Design review of the part built by this model. Coordinates are the model's own, in mm. A direction names the side the tool comes from. Coordinates: 2 decimals unless noted, no trailing zeros. Order: outer loops, then holes, each group sorted by start corner. A loop starts at its lowest first (then second) coordinate and runs counter-clockwise, first axis right, second up.
from build123d import *

# Parameters (mm, degrees)
CROQUIS2_W                   = 50
CROQUIS2_H                   = 70
SALIENTE_EXTRUIR1_DEPTH      = 10
SALIENTE_EXTRUIR2_DEPTH      = 30
SALIENTE_EXTRUIR2_DEPTH_BACK = 30
CROQUIS4_R                   = 2.5
CROQUIS5_R                   = 10
SALIENTE_EXTRUIR3_DEPTH      = 5
CROQUIS6_R                   = 2.5
SALIENTE_EXTRUIR4_DEPTH      = 10
REDONDEO1_R                  = 2


with BuildPart() as part:
    # Croquis2 → Saliente-Extruir1 (new body)
    with BuildSketch(Plane(origin=(0, 0, 0), x_dir=(1, 0, 0), z_dir=(0, 1, 0))):
        Rectangle(CROQUIS2_W, CROQUIS2_H)
    extrude(amount=SALIENTE_EXTRUIR1_DEPTH)

    # Croquis4 → Saliente-Extruir2 (add, two sides: drawn at the far end of the back side and taken through both)
    with BuildSketch(Plane(origin=(0, 0, 0), x_dir=(0, 0, -1), z_dir=(1, 0, 0)).offset(-SALIENTE_EXTRUIR2_DEPTH_BACK)):
        with Locations((-29.646809276, 0)):
            Circle(CROQUIS4_R)
    extrude(amount=SALIENTE_EXTRUIR2_DEPTH + SALIENTE_EXTRUIR2_DEPTH_BACK)

    # Croquis5 → Saliente-Extruir3 (add)
    with BuildSketch(Plane(origin=(30, 0, 0), x_dir=(0, 0, -1), z_dir=(1, 0, 0))):
        with Locations((-29.646809276, 0)):
            Circle(CROQUIS5_R)
    saliente_extruir3 = extrude(amount=SALIENTE_EXTRUIR3_DEPTH)

    # Simetría1: Saliente-Extruir3 across plane
    add(saliente_extruir3.mirror(Plane(origin=(0, 0, 0), x_dir=(0, 0, 1), z_dir=(1, 0, 0))))

    # Croquis6 → Saliente-Extruir4 (add)
    with BuildSketch(Plane.XZ):
        with Locations(Location((0, -30, 0), (0, 0, 270))):
            Circle(CROQUIS6_R)
    extrude(amount=SALIENTE_EXTRUIR4_DEPTH)

    # Redondeo1
    redondeo1_edges = [part.edges().sort_by_distance(p)[0] for p in [
        (0, -10, -27.5),
    ]]
    fillet(redondeo1_edges, radius=REDONDEO1_R)


solid = part.part
1. For faces 4 (the flat face through (0, 0, 34)), 5 (the cylindrical face through (32.465, 0.44, 39.637)), 6 (the flat face through (-30, -2.1, 27.6)), 7 (the flat face through (0, 5, 35)), list the 3-axis set-ups (+Z, -Z, +X, -X, +Y, -Y) from which the entire face can be reached by the end or side of a thin tool; tool diameter is ignored.
2. Add section B-B (x = 8). Give the boundary of the cut face in (y, z), and give its area (3 significant figures).
3. To check wall thickness, follow line 1 (X direction, y = 5.75, z = 30); line 2 (X direction, y = -3, z = 29); line 3 (Y direction, x = -15, z = 9.5). State the ranges of each line that lie inside material, in increasing order.
4. Insertion check: pin 1 (15 mm diameter, centred on x = -3.5, z = -17.5, fed in from -Y); pin 2 (11 mm diameter, centred on x = -10.5, y = 3.5, fed in from +Z); pin 3 (3 mm diameter, centred on y = 3.5, z = 7, fed in from +X). Each pin has a flat end and moves straight along its axis. Give the tip position at first contact, or say it passes through.
5. Mouldability with a two-part tool opening along Z and no side actions: class faces 1 (the cylindrical face through (0.1, -3.9, -27.5)), 2 (the flat face through (0, 5, -35)), 3 (the flat face through (25, 5, 0)) as pulls with the +Z half, pulls with the -Z half, needs draft (parallel to the pull), parting line crosses it, or undercut.
6. Add section D-D (z = -8). Give the boundary of the cut face in (x, y).
7. Add section A-A (y = -1). Give the boundary of the cut face in (x, z), and give its area (3 significant figures).
8. Add section C-C (y = 6.75). Give the boundary of the cut face in (x, z), and give its area (3 significant figures).
Solution:
1. face 4: +Z, -Y
1. face 5: +X
1. face 6: none
1. face 7: +Z, +Y, -Y
2. outline: (0, -35) - (10, -35) - (10, 35) - (0, 35) - (0, 32.15) arc R2.5 ccw to (0, 27.15) - close
2. area: 710 mm2
3. line 1: x = -35 to -30, -25 to 25, 30 to 35
3. line 2: x = -35 to -30, 30 to 35
3. line 3: y = 0 to 10
4. pin 1: stops at y = 0
4. pin 2: stops at z = 35
4. pin 3: stops at x = 25
5. face 1: undercut
5. face 2: pulls with the -Z half
5. face 3: needs draft
6. outline: (-25, 0) - (25, 0) - (25, 10) - (-25, 10) - close
7. outline: (-35, 19.7) - (-30, 19.7) - (-30, 27.36) - (30, 27.36) - (30, 19.7) - (35, 19.7) - (35, 39.6) - (30, 39.6) - (30, 31.94) - (-30, 31.94) - (-30, 39.6) - (-35, 39.6) - close; circle Ø5 at (0, -30)
7. area: 494 mm2
8. outline: (-35, 22.27) - (-30, 22.27) - (-30, 37.02) - (-35, 37.02) - close; (-25, -35) - (25, -35) - (25, 35) - (-25, 35) - close; (30, 22.27) - (35, 22.27) - (35, 37.02) - (30, 37.02) - close
8. area: 3,650 mm2
